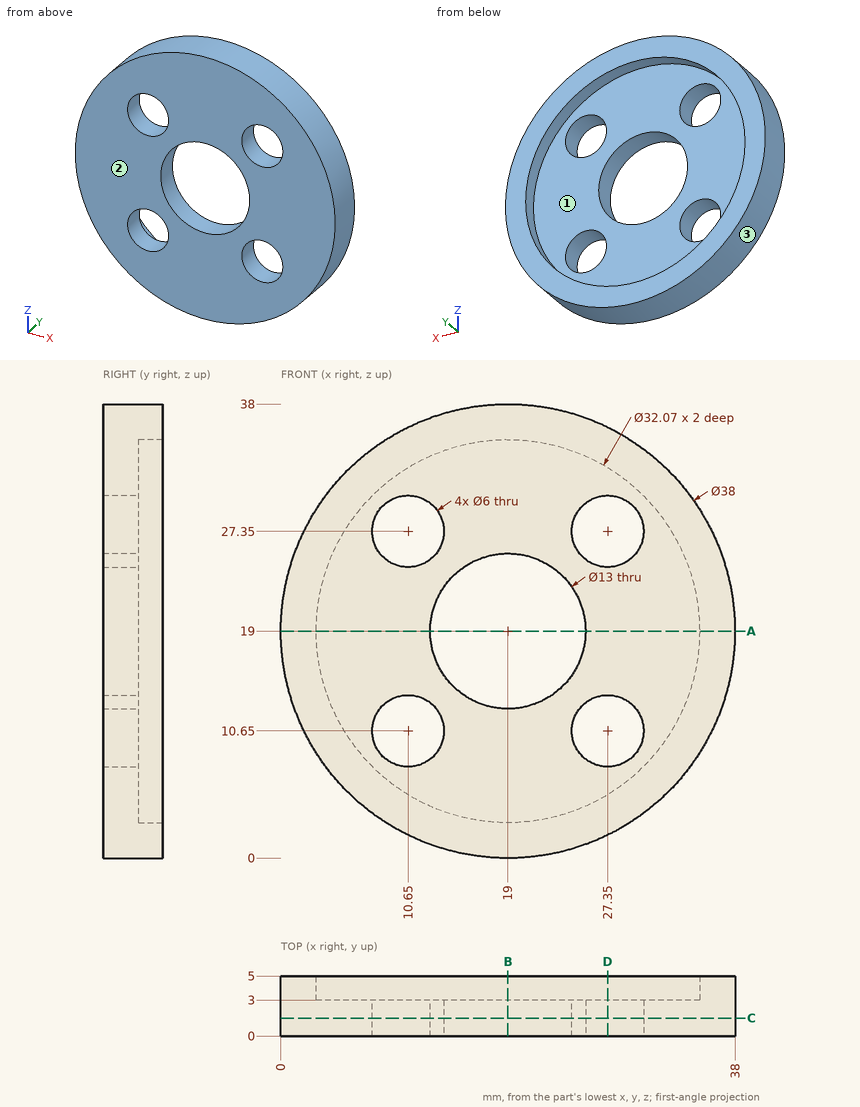
Here's the drawing with two shaded views (mm, measured from the low corner). I have some questions. Coordinates: 2 decimals unless noted, no trailing zeros. Write each loop counter-clockwise with the first axis right and the second up, starting at its lowest first coordinate (ties: lowest second). Pieces come first, ordered by that corner, then holes. Notation, with made-up numbers: (-29.75, -38) -> (27.25, -38) arc R20 ccw to (27.25, -28) -> close; hole circle Ø7 at (48.5, 43.5). An arc over 180 degrees is marked (long way). Write item = value, one per line. Start each with the question number.
(1) I want a section at B-B (x = 19). Please give me the cut outline in (y, z) (3 decimals).
(2) I want a section at D-D (x = 27.35). Please give me the cut outline in (y, z), plus the area to 3 significant figures.
(3) I need wall thicknesses on line 1 (X direction, y = 0.45, z = 30); line 2 (X direction, y = 1.1, z = 10.65); line 3 (X direction, y = 2.15, z = 25). Which ranges of each line are inside material? Lowest first, please. Write a range as [from, to].
(4) We'd pull the mould along X, two halves only. Please class the marked faces 1, 2 and 3: released by +X, released by -X, zero draft, split by the parting line, or undercut.
(5) I want a section at C-C (y = 1.5). Please give me the cut outline in (x, z), plus the area to 3 significant figures.
(6) I want a section at A-A (z = 19). Please give me the cut outline in (x, y) (3 decimals).
(7) Will these pins go through, and if not, where does the flat tip stop? pin 1 (1 mm diameter, centred on x = 27.5, z = 19, fed in from -Y); pin 2 (1 mm diameter, centred on x = 19.5, y = 1.5, fed in from +Z); pin 3 (3 mm diameter, centred on x = 10.5, y = 2.5, fed in from +Z); pin 4 (9.5 mm diameter, centred on x = 16.5, z = 23, fed in from +Y).
Result set:
q1.outline = (0, 0) -> (5, 0) -> (5, 2.965) -> (3, 2.965) -> (3, 12.5) -> (0, 12.5) -> close; (0, 25.5) -> (3, 25.5) -> (3, 35.035) -> (5, 35.035) -> (5, 38) -> (0, 38) -> close
q2.outline = (0, 1.93) -> (5, 1.93) -> (5, 5.31) -> (3, 5.31) -> (3, 7.65) -> (0, 7.65) -> close; (0, 13.65) -> (3, 13.65) -> (3, 24.35) -> (0, 24.35) -> close; (0, 30.35) -> (3, 30.35) -> (3, 32.69) -> (5, 32.69) -> (5, 36.07) -> (0, 36.07) -> close
q2.area = 79.9 mm2
q3.line_1 = [3.51, 9.24], [12.06, 25.94], [28.76, 34.49]
q3.line_2 = [1.93, 7.65], [13.65, 24.35], [30.35, 36.07]
q3.line_3 = [0.97, 8.79], [12.51, 16.5], [21.5, 25.49], [29.21, 37.03]
q4.face_1 = undercut
q4.face_2 = zero draft
q4.face_3 = split by the parting line
q5.outline = circle Ø38 at (19, 19); hole circle Ø6 at (10.65, 10.65); hole circle Ø6 at (10.65, 27.35); hole circle Ø13 at (19, 19); hole circle Ø6 at (27.35, 10.65); hole circle Ø6 at (27.35, 27.35)
q5.area = 888 mm2
q6.outline = (0, 0) -> (12.5, 0) -> (12.5, 3) -> (2.965, 3) -> (2.965, 5) -> (0, 5) -> close; (25.5, 0) -> (38, 0) -> (38, 5) -> (35.035, 5) -> (35.035, 3) -> (25.5, 3) -> close
q7.pin_1 = 0
q7.pin_2 = 38
q7.pin_3 = 36.66
q7.pin_4 = 3
